Part model, mm, in its own coordinate system. A direction names the side the tool comes from. Round coordinates to 2 decimals unless told otherwise and drop trailing zeros. Loops run counter-clockwise (first coordinate to the right, second up) from the corner with the lowest first, then second, coordinate; pieces in that order, holes last.
1) Mould opens along X. For faces 1 (the cylindrical face through (-0.751, 1.267, 8.385)), 2 (the flat face through (-15, 25, 0)), 3 (the flat face through (0, 25, 9)), 4 (the flat face through (0, 50, 0)) say: +X half, -X half, draft (parallel to the pull), parting line (faces both ways), or undercut.
2) 3-axis set-ups, long thin cutter, end or side, ignore diameter. For faces 5 (the flat face through (6.9, 25.5, 4)), 6 (the cylindrical face through (0, 25.5, 3.5)), 7 (the flat face through (0, 25, 11.5)): which of +Z, -Z, +X, -X, +Y, -Y reach the whole face in a straight line?
3) Probe line 1 (Y direction, x = 4, z = -4.25); line 2 (X direction, y = 37, z = 0.5); line 3 (Z direction, x = -12.25, y = 45). List the from-to ranges inside material, lowest first.
4) Band-saw the part on B-B, the plane y = 4.5. Write the cut outline in (x, z).
5) Band-saw the part on C-C, the plane x = 9.75. Write the cut outline in (y, z), then the cut area to 3 significant figures.
6) Band-saw the part on A-A, the plane z = -1. Write the cut outline in (x, y).
7) Band-saw the part on D-D, the plane z = 6. Write the cut outline in (x, y), then the cut area to 4 significant figures.
from build123d import *

# Parameters (mm, degrees)
SKETCH1_W           = 30
SKETCH1_H           = 23
BOSS_EXTRUDE1_DEPTH = 50
CUT_EXTRUDE2_START  = 2.5
SKETCH1_5_W         = 25
SKETCH1_5_H         = 18
CUT_EXTRUDE2_DEPTH  = 45
BOSS_EXTRUDE3_START = 25
SKETCH1_6_W         = 25
SKETCH1_6_H         = 18
BOSS_EXTRUDE3_DEPTH = 1
CUT_EXTRUDE3_START  = 21.5
SKETCH2_R           = 2.5
CUT_EXTRUDE3_DEPTH  = 26
SKETCH4_W           = 25
SKETCH4_H           = 5
CUT_EXTRUDE4_DEPTH  = 1


with BuildPart() as part:
    # Sketch1 → Boss-Extrude1 (new body)
    with BuildSketch(Plane(origin=(0, 0, 0), x_dir=(1, 0, 0), z_dir=(0, 1, 0))):
        Rectangle(SKETCH1_W, SKETCH1_H)
    extrude(amount=BOSS_EXTRUDE1_DEPTH)

    # Sketch1<5> → Cut-Extrude2 (cut)
    with BuildSketch(Plane(origin=(0, 0, 0), x_dir=(1, 0, 0), z_dir=(0, 1, 0)).offset(CUT_EXTRUDE2_START)):
        Rectangle(SKETCH1_5_W, SKETCH1_5_H)
    extrude(amount=CUT_EXTRUDE2_DEPTH, mode=Mode.SUBTRACT)

    # Sketch1<6> → Boss-Extrude3 (add)
    with BuildSketch(Plane(origin=(0, 0, 0), x_dir=(1, 0, 0), z_dir=(0, 1, 0)).offset(BOSS_EXTRUDE3_START)):
        Rectangle(SKETCH1_6_W, SKETCH1_6_H)
    extrude(amount=BOSS_EXTRUDE3_DEPTH)

    # Sketch2 → Cut-Extrude3 (cut)
    with BuildSketch(Plane(origin=(0, 47.5, 0), x_dir=(-1, 0, 0), z_dir=(0, -1, 0)).offset(CUT_EXTRUDE3_START)):
        with Locations(Location((0, -6, 0), (0, 0, 270))):
            Circle(SKETCH2_R)
    extrude(amount=CUT_EXTRUDE3_DEPTH, mode=Mode.SUBTRACT)

    # Sketch4 → Cut-Extrude4 (cut)
    with BuildSketch(Plane(origin=(0, 26, 0), x_dir=(1, 0, 0), z_dir=(0, 1, 0))):
        with Locations((0, -6.5)):
            Rectangle(SKETCH4_W, SKETCH4_H)
    extrude(amount=-CUT_EXTRUDE4_DEPTH, mode=Mode.SUBTRACT)


solid = part.part
Reported:
1. face 1: undercut
1. face 2: -X half
1. face 3: undercut
1. face 4: draft
2. face 5: none
2. face 6: -Y
2. face 7: +Z, +X, -X, +Y, -Y
3. line 1: y = 0 to 2.5, 25 to 26, 47.5 to 50
3. line 2: x = -15 to -12.5, 12.5 to 15
3. line 3: z = -11.5 to -9, 9 to 11.5
4. outline: (-15, -11.5) - (15, -11.5) - (15, 11.5) - (-15, 11.5) - close; hole (-12.5, -9) - (12.5, -9) - (12.5, 9) - (-12.5, 9) - close
5. outline: (0, -11.5) - (50, -11.5) - (50, 11.5) - (0, 11.5) - close; hole (2.5, -9) - (25, -9) - (25, 4) - (26, 4) - (26, -9) - (47.5, -9) - (47.5, 9) - (2.5, 9) - close
5. area: 353 mm2
6. outline: (-15, 0) - (15, 0) - (15, 50) - (-15, 50) - close; hole (-12.5, 2.5) - (12.5, 2.5) - (12.5, 25) - (-12.5, 25) - close; hole (-12.5, 26) - (12.5, 26) - (12.5, 47.5) - (-12.5, 47.5) - close
7. outline: (-15, 0) - (-2.5, 0) - (-2.5, 2.5) - (-12.5, 2.5) - (-12.5, 47.5) - (12.5, 47.5) - (12.5, 2.5) - (2.5, 2.5) - (2.5, 0) - (15, 0) - (15, 50) - (-15, 50) - close
7. area: 362.5 mm2
